Autodesk Inventor part; units mm, degrees
ref_plane "YZ Plane" through (0, 0, 0) normal (1, 0, 0) x (0, 1, 0)
ref_plane "XZ Plane" through (0, 0, 0) normal (0, 1, 0) x (-1, 0, 0)
ref_plane "XY Plane" through (0, 0, 0) normal (0, 0, 1) x (1, 0, 0)
sketch "Sketch1" plane through (0, 0, 0) normal (0, 0, 1) x (1, 0, 0)
  line L0 (-13.3613, 31.5734) -> (9.3717, 31.5734)
  line L1 (9.3717, 31.5734) -> (9.3717, -35.1016)
  line L2 (9.3717, -35.1016) -> (-13.3613, -35.1016)
  line L3 (-13.3613, -35.1016) -> (-13.3613, 31.5734)
  line L4 (10.1591, 32.3608) -> (-14.1487, 32.3608)
  line L5 (-14.1487, 32.3608) -> (-14.1487, -35.889)
  line L6 (-14.1487, -35.889) -> (10.1591, -35.889)
  line L7 (10.1591, -35.889) -> (10.1591, 32.3608)
  line L8 (8.5843, 30.786) -> (-12.5739, 30.786)
  line L9 (-12.5739, 30.786) -> (-12.5739, -34.3142)
  line L10 (-12.5739, -34.3142) -> (8.5843, -34.3142)
  line L11 (8.5843, -34.3142) -> (8.5843, 30.786)
  point P0 (0, 0)
  dimension "d0" = 22.733
  dimension "d1" = 66.675
  dimension "d2" = 0.7874
  dimension "d3" = 0.7874
extrude "Extrusion1" add sketch "Sketch1" along normal blind 1.5875 contours L0 L1 L2 L3 | L7 L6 L5 L4
sketch "Sketch3" plane through (0, 0, 1.5875) normal (0, 0, 1) x (1, 0, 0)
  line L0 (-14.1487, 32.3608) -> (10.1591, 32.3608)
  line L1 (10.1591, 32.3608) -> (10.1591, -35.889)
  line L2 (10.1591, -35.889) -> (-14.1487, -35.889)
  line L3 (-14.1487, -35.889) -> (-14.1487, 32.3608)
  point P0 (0, 0)
extrude "Extrusion2" add sketch "Sketch3" along normal blind 1.5875
sketch "Sketch4" plane through (0, 0, 1.5875) normal (0, 0, -1) x (-1, 0, 0)
  line L0 (1.1699, -25.422) -> (5.9324, -25.422)
  line L1 (5.9324, -25.422) -> (5.9324, -30.1845)
  line L2 (5.9324, -30.1845) -> (1.1699, -30.1845)
  line L3 (1.1699, -30.1845) -> (1.1699, -25.422)
  point P0 (0, 0)
  dimension "d10" = 4.7625
  dimension "d11" = 4.7625
extrude "Extrusion3" add sketch "Sketch4" along normal blind 0.508
properties part number "YagiCan"
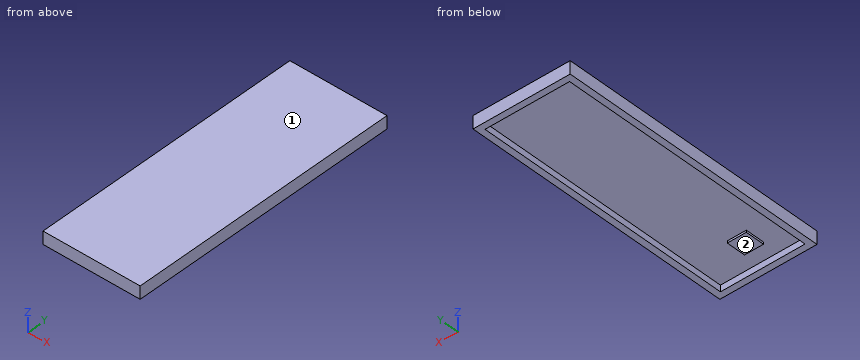
Geometry check sheet. Reference: the model listing, model coordinates, mm. Face numbers are marked on the shaded views. Give positions to 0.01 mm unless a question says otherwise; leave off trailing zeros. Write each loop counter-clockwise with the first axis right and the second up, starting at its lowest first coordinate (ties: lowest second). Pieces come first, ordered by that corner, then holes.
1) Cross-section at A-A (x = -3.5). Record the boundary of the cut face in (y, z) (1 decimal).
Values follow:
outline: (-35.9, 0) - (-34.3, 0) - (-34.3, 1.6) - (-30.2, 1.6) - (-30.2, 1.1) - (-25.4, 1.1) - (-25.4, 1.6) - (30.8, 1.6) - (30.8, 0) - (32.4, 0) - (32.4, 3.2) - (-35.9, 3.2) - close
2) Go/stop test with flat-tipped pins: pin 1 Ø1.4 at (x, y) = (-4, -28.5) entering from -Z; pin 2 Ø1 at (x, y) = (3, -0.5) entering from -Z. Record where each tip stops, or that it passes through.
Values follow:
pin 1: stops at z = 1.08
pin 2: stops at z = 1.59
3) Cross-section at B-B (y = 25.5). Record the boundary of the cut face in (x, z) (1 decimal), plus the area to 3 significant figures.
Values follow:
outline: (-14.1, 0) - (-12.6, 0) - (-12.6, 1.6) - (8.6, 1.6) - (8.6, 0) - (10.2, 0) - (10.2, 3.2) - (-14.1, 3.2) - close
area: 43.6 mm2
4) Thickness scan on line 1 (Y direction, x = 7, z = 0.3); line 2 (X direction, y = -15, z = 0.6); line 3 (Z direction, x = -8, y = -15) (1 decimal). Record the ranges inside material, lowest first.
Values follow:
line 1: y = -35.89 to -34.31, 30.79 to 32.36
line 2: x = -14.15 to -12.57, 8.58 to 10.16
line 3: z = 1.6 to 3.2
5) Release check for a two-part mould opening along X. For the marked faces 1 and 2 record: released by +X, released by -X, zero draft, split by the parting line, or undercut.
Values follow:
face 1: zero draft
face 2: undercut
6) Cross-section at C-C (x = -10.5). Record the boundary of the cut face in (y, z) (1 decimal), plus the area to 3 significant figures.
Values follow:
outline: (-35.9, 0) - (-34.3, 0) - (-34.3, 1.6) - (30.8, 1.6) - (30.8, 0) - (32.4, 0) - (32.4, 3.2) - (-35.9, 3.2) - close
area: 113 mm2
7) Cross-section at D-D (y = -28). Record the boundary of the cut face in (x, z) (1 decimal).
Values follow:
outline: (-14.1, 0) - (-12.6, 0) - (-12.6, 1.6) - (-5.9, 1.6) - (-5.9, 1.1) - (-1.2, 1.1) - (-1.2, 1.6) - (8.6, 1.6) - (8.6, 0) - (10.2, 0) - (10.2, 3.2) - (-14.1, 3.2) - close
